Input: part model. Units: mm. Frame: model coordinates. A direction names the side the tool comes from. Coordinates: 2 decimals unless noted, no trailing zeros. Order: outer loops, then holes, each group sorted by start corner. A loop starts at its lowest first (then second) coordinate and runs counter-clockwise, first axis right, second up.
Autodesk Inventor part; units mm, degrees
ref_plane "YZ Plane" through (0, 0, 0) normal (1, 0, 0) x (0, 1, 0)
ref_plane "XZ Plane" through (0, 0, 0) normal (0, 1, 0) x (-1, 0, 0)
ref_plane "XY Plane" through (0, 0, 0) normal (0, 0, 1) x (1, 0, 0)
sketch "Sketch1" plane through (0, 0, 0) normal (0, 0, 1) x (1, 0, 0)
  line L0 (-1.3333, 0) -> (40, 0)
  line L1 (40, 0) -> (40, 3)
  line L2 (40, 3) -> (16, 3)
  line L3 (16, 3) -> (15.3864, 3)
  line L4 (15.3864, 3) -> (0, 3)
  line L5 (0, 3) -> (0, 5)
  line L6 (0, 5) -> (-6, 5)
  line L7 (-6, 5) -> (-6, 2.8868)
  line L8 (-6, 2.8868) -> (-3, 2.8868)
  line L9 (-3, 2.8868) -> (-1.3333, 0)
  line L10 (-15.2, 0) -> (49.2, 0)
  line L11 (0, -1) -> (0, 6)
  line L12 (16, 3) -> (0, 3) construction
  dimension "d1" = 24
  dimension "d2" = 0.6136
  dimension "d3" = 6
  dimension "d4" = 3
  dimension "d5" = 60
  dimension "d6" = 6
  dimension "d7" = 6
  dimension "d8" = 5.7735
  dimension "d9" = 10
  dimension "d26" = 40
revolve "Body" add sketch "Sketch1" angle 360 about axis through (-1.3333, 0, 0) along (1, 0, 0)
sketch "Sketch2" plane through (-6, 0, 0) normal (-1, 0, 0) x (0, 0, 1)
  circle A0 centre (0, 0) radius 2.8868
  line L0 (0, -7) -> (0, 7)
  line L1 (-7, 0) -> (7, 0)
  line L2 (2.8868, 0) -> (1.4434, -2.5)
  line L3 (1.4434, -2.5) -> (-1.4434, -2.5)
  line L4 (-1.4434, -2.5) -> (-2.8868, 0)
  line L5 (-2.8868, 0) -> (-1.4434, 2.5)
  line L6 (-1.4434, 2.5) -> (1.4434, 2.5)
  line L7 (1.4434, 2.5) -> (2.8868, 0)
extrude "Slot" add sketch "Sketch2" against normal up to next contours L7 A0 | A0 L2 | L6 L0 A0 | A0 L0 L3 | L0 L6 A0 | A0 L3 L0 | L4 A0 | A0 L5
fillet "Fillet1" radius 0.6 1 edges at (-6, -5, 0)
thread "Thread"
equation "\"d1\" = GEL"
equation "\"d3\" = KOH"
equation "\"d4\" = INTI"
equation "\"d6\" = GD"
equation "\"d7\" = BDM"
equation "\"d8\" = 1.1547 * SW"
equation "\"d9\" = KOD"
equation "\"d26\" = NLG"
equation "\"d17\" = RR"
equation "\"d13\" = GEL"
equation "\"GD\" = 6"
equation "\"NLG\" = 40"
equation "\"GEL\" = 24"
equation "\"KOD\" = 10"
equation "\"KOH\" = 6"
equation "\"INTI\" = 3"
equation "\"GAL\" = 0.61345 * PTC"
equation "\"GUL\" = 0.61345 * PTC"
equation "\"BDM\" = NND"
equation "\"SW\" = 5"
equation "\"RR\" = 0.6"
equation "\"SPD\" = NND - 1.2269 * PTC"
equation "\"R\" = 0.1"
equation "\"TOA\" = 30deg"
equation "\"GD1\" = THREADDIA - 1.2269 * PTC"
equation "\"THREADDIA\" = 6"
equation "\"FAWI\" = 45deg"
equation "\"PTC\" = 1"
equation "\"NND\" = 6"
equation "\"E0\" = 1.155 * SW"
equation "\"d38\" = 55deg"
equation "\"Sketch4_Pitch\" = 1"
properties part number "ISO 4762 - M6 x 40" material "Stainless Steel, 440C"
Item 1: Pin query (flat end, axial travel): pin 1 Ø3 at (x, y) = (15.5, -2) entering from +Z; pin 2 Ø1.5 at (x, z) = (31, 0.5) entering from +Y. Return the tip coordinate at first contact, or that it passes through.
Response values:
pin 1: stops at z = 2.96
pin 2: stops at y = 3
Item 2: Ray query, probe 1 along X at (y, z) = (-1.75, 1); probe 2 along X at (y, z) = (-3.25, 1); probe 3 along Z at (x, y) = (38, 0). Return the intervals inside material, ascending.
Response values:
probe 1: x = -2.5 to 40
probe 2: x = -6 to 0
probe 3: z = -3 to 3
Item 3: Cut plane A-A on x = 2. Return loops of the section in (y, z), then the cut area to 3 significant figures.
Response values:
outline: circle Ø6 at (0, 0)
area: 28.3 mm2
Item 4: Draft query along Z for faces 1 (the face through (-4.411, -1.233, 2.175)), 2 (the face through (40, 0, 0)), 3 (the face through (20, -3, 0)). Return one class per face: pulls with the +Z half, pulls with the -Z half, needs draft (parallel to the pull), parting line crosses it, or undercut.
Response values:
face 1: undercut
face 2: needs draft
face 3: parting line crosses it
Item 5: Access query for faces 4 (the face through (-2.74, -1.08, 4.88)), 5 (the face through (0, 3.3, 0.1)), 6 (the face through (-4.411, 1.233, -2.175)). Directions: +Z, -Z, +X, -X, +Y, -Y. A direction counts if a zero-diameter tool reaches every point of the face in a straight line with its end or side. Return the directions, or none.
Response values:
face 4: +X, -X
face 5: +X
face 6: -X
